from build123d import *

# Parameters (mm, degrees)
F0_W      = 28
F0_H      = 16
F1_DEPTH  = 5
F2_R      = 1.2
F3_DEPTH  = 5.001
F4_W      = 16
F4_H      = 20
F5_DEPTH  = 25
F6_R      = 4
F7_DEPTH  = 16.001
F8_W      = 16
F8_H      = 7.6
F9_DEPTH  = 10
F10_R     = 2
F11_DEPTH = 20.001
F12_DEPTH = 15
F13_R     = 5
F14_R     = 5


with BuildPart() as f1:
    # F0 (on Top) → F1 (new body)
    with BuildSketch(Plane.XY):
        with Locations((14, 8)):
            Rectangle(F0_W, F0_H)
    extrude(amount=F1_DEPTH)

    # F2 (on face) → F3 (cut, through all)
    with BuildSketch(Plane.XY.offset(5)):
        with Locations((12.52, 13.25)):
            Circle(F2_R)
        with Locations((3, 13.25)):
            Circle(F2_R)
    extrude(amount=-F3_DEPTH, mode=Mode.SUBTRACT)

    # F4 (on face) → F5 (join)
    with BuildSketch(Plane(origin=(0, 0, 0), x_dir=(0, -1, 0), z_dir=(-1, 0, 0))):
        with Locations((-8, 2.5)):
            Rectangle(F4_W, F4_H)
    extrude(amount=F5_DEPTH)

    # F6 (on face) → F7 (cut, through all)
    with BuildSketch(Plane(origin=(0, 16, 0), x_dir=(-1, 0, 0), z_dir=(0, 1, 0))):
        with Locations((10, 2.5)):
            Circle(F6_R)
    extrude(amount=-F7_DEPTH, mode=Mode.SUBTRACT)

    # F8 (on face) → F9 (cut)
    with BuildSketch(Plane(origin=(-25, 0, 0), x_dir=(0, -1, 0), z_dir=(-1, 0, 0))):
        with Locations((-8, 2.5)):
            Rectangle(F8_W, F8_H)
    extrude(amount=-F9_DEPTH, mode=Mode.SUBTRACT)

    # F10 (on face) → F11 (cut, through all)
    with BuildSketch(Plane.XY.offset(12.5)):
        with Locations((-21, 9.280348)):
            Circle(F10_R)
    extrude(amount=-F11_DEPTH, mode=Mode.SUBTRACT)

    # F8 (on face) → F12 (cut)
    with BuildSketch(Plane(origin=(-25, 0, 0), x_dir=(0, -1, 0), z_dir=(-1, 0, 0))):
        with Locations((-8, 2.5)):
            Rectangle(F8_W, F8_H)
    extrude(amount=-F12_DEPTH, mode=Mode.SUBTRACT)

    # F13
    f13_edges = [f1.edges().sort_by_distance(p)[0] for p in [
        (0, 8, 12.5),
    ]]
    fillet(f13_edges, radius=F13_R)

    # F14
    f14_edges = [f1.edges().sort_by_distance(p)[0] for p in [
        (0, 8, -7.5),
    ]]
    fillet(f14_edges, radius=F14_R)


solid = f1.part
Here's how the part is built. I have some questions about the finished solid (model axes, mm). A direction names the side the tool comes from. Coordinates: 2 decimals unless noted, no trailing zeros. Order: outer loops, then holes, each group sorted by start corner. A loop starts at its lowest first (then second) coordinate and runs counter-clockwise, first axis right, second up.
Item 1: If we section it at C-C on z = 2.5: List the corners of the cut face in (x, y) for me.
Result sheet:
outline: (-6, 0) - (28, 0) - (28, 16) - (-6, 16) - close; hole circle Ø2.4 at (3, 13.25); hole circle Ø2.4 at (12.52, 13.25)
Item 2: If we section it at D-D on y = 5.5: List the corners of the cut face in (x, z) for me, plus the area to 3 significant figures.
Result sheet:
outline: (-25, -7.5) - (-5, -7.5) arc R5 ccw to (0, -2.5) - (0, 0) - (28, 0) - (28, 5) - (0, 5) - (0, 7.5) arc R5 ccw to (-5, 12.5) - (-25, 12.5) - (-25, 6.3) - (-11.25, 6.3) arc R4 cw (long way) to (-11.25, -1.3) - (-25, -1.3) - close
area: 490 mm2
Item 3: If we section it at A-A on x = 12.52: List the corners of the cut face in (y, z) for me, plus the area to 3 significant figures.
Result sheet:
outline: (0, 0) - (12.05, 0) - (12.05, 5) - (0, 5) - close; (14.45, 0) - (16, 0) - (16, 5) - (14.45, 5) - close
area: 68.0 mm2
Item 4: I need wall thicknesses on line 1 (Y direction, x = 3, z = 2.95); line 2 (Z direction, x = 22.5, y = 6); line 3 (X direction, y = 12.25, z = 4.25). Which ranges of each line are inside material? Lowest first, please.
Result sheet:
line 1: y = 0 to 12.05, 14.45 to 16
line 2: z = 0 to 5
line 3: x = -6.4 to 2.34, 3.66 to 11.86, 13.18 to 28
Item 5: If we mould it in two halves opening along X, with no side actions, what happens to faces 1 (the face through (28, 8, 2)), 2 (the face through (-15, 8, 12.5)), 3 (the face through (12.26, 12.08, 2.54))? For each: +X half, -X half, draft (parallel to the pull), parting line (faces both ways), or undercut.
Result sheet:
face 1: +X half
face 2: draft
face 3: undercut
Item 6: If we section it at B-B on y = 13.25: List the corners of the cut face in (x, z) for me, plus the area to 3 significant figures.
Result sheet:
outline: (-25, -7.5) - (-5, -7.5) arc R5 ccw to (0, -2.5) - (0, 0) - (1.8, 0) - (1.8, 5) - (0, 5) - (0, 7.5) arc R5 ccw to (-5, 12.5) - (-25, 12.5) - (-25, 6.3) - (-11.25, 6.3) arc R4 cw (long way) to (-11.25, -1.3) - (-25, -1.3) - close; (4.2, 0) - (11.32, 0) - (11.32, 5) - (4.2, 5) - close; (13.72, 0) - (28, 0) - (28, 5) - (13.72, 5) - close
area: 466 mm2
Item 7: For faces 4 (the face through (0, 8, -1)), 5 (the face through (14, 8, 5)), 6 (the face through (-18, 8, -1.3)), which set-ups out of +Z, -Z, +X, -X, +Y, -Y let a thin tool reach every point of the face, with its end or its side?
Result sheet:
face 4: -Z, +X, +Y, -Y
face 5: +Z, +X, +Y, -Y
face 6: -X, +Y, -Y
Item 8: For P1, Ø0.8, axis at y = 7.5, z = 6.5, coming from the +X side; P2, Ø3.5, axis at x = -21, y = 9.28, coming from the +Z side; P3, Ø8, axis at x = 19, y = 5.5, coming from the -Z side; P4, Ø8, axis at x = 12, y = 11.5, coming from the +Z side, each with a flat end and sliding along its axis, tell me the tip position at first contact or that it passes through.
Result sheet:
P1: stops at x = 0
P2: passes through
P3: stops at z = 0
P4: stops at z = 5
